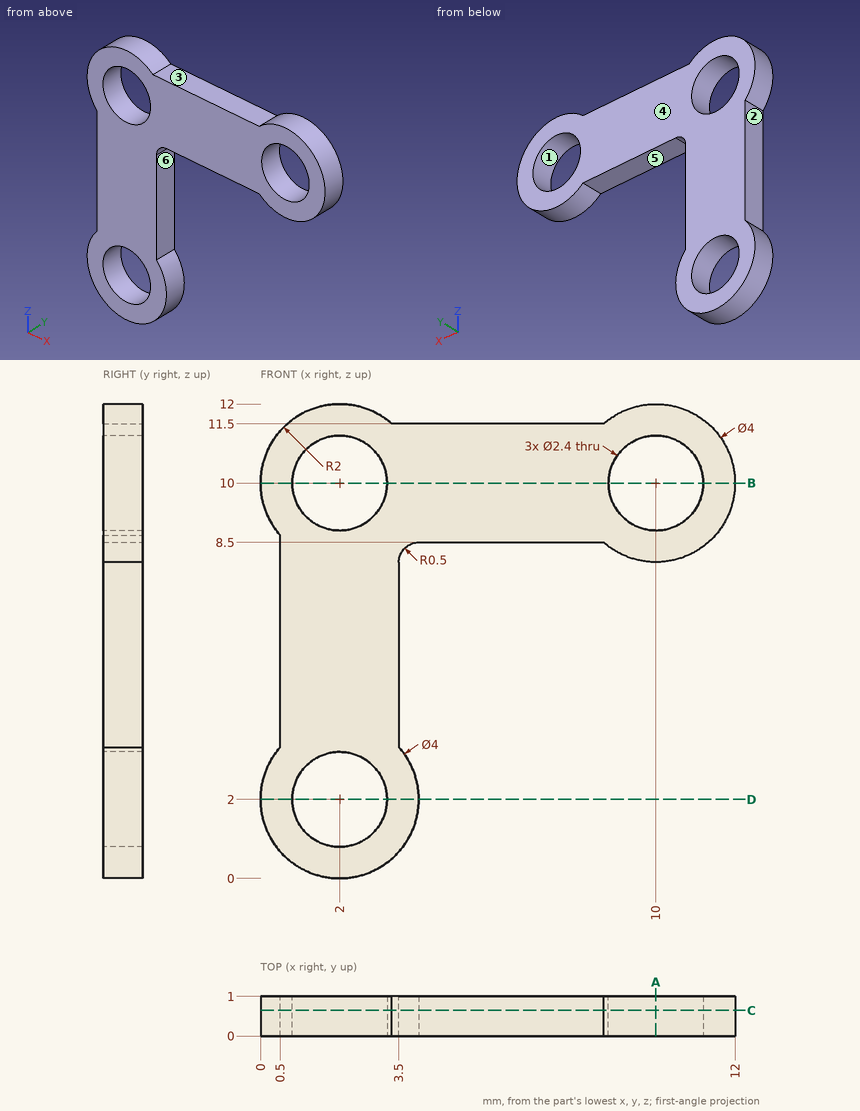
Geometry check sheet. Reference: drawing and pictorial views, mm from the part's lowest x, y, z. A direction names the side the tool comes from. Round coordinates to 2 decimals unless told otherwise and drop trailing zeros. Order: outer loops, then holes, each group sorted by start corner. A loop starts at its lowest first (then second) coordinate and runs counter-clockwise, first axis right, second up. Notation, with made-up numbers: M -21,-13 L -3,-13 A14 ccw -3,-8 Z; hole C 19.5,-1 d3. An arc over 180 degrees is marked long. Answer as CSV lines item,"result".
1) Gauge pin test, flat ends, axial feed: pin 1 Ø3 at (x, z) = (2, 2) entering from -Y; pin 2 Ø2 at (x, z) = (10, 10) entering from +Y. Record the tip position at first contact, or that the pin passes through.
Entries:
pin 1,"y = 0"
pin 2,"through"
2) Tool access check on the marked faces 1, 2 and 3. Record the directions out of +Z, -Z, +X, -X, +Y, -Y that give a thin tool (end or side, any length) a straight path to the whole face; none if there is none.
Entries:
face 1,"+Y, -Y"
face 2,"-X, +Y, -Y"
face 3,"+Z, +Y, -Y"
3) Sectioned sample at C-C on y = 0.65. Record the cut outline in (x, z).
Entries:
outline,"M 0.5,3.32 A2 ccw long 3.5,3.32 L 3.5,8 A0.5 cw 4,8.5 L 8.68,8.5 A2 ccw long 8.68,11.5 L 3.32,11.5 A2 ccw 0.5,8.68 Z; hole C 2,2 d2.4; hole C 2,10 d2.4; hole C 10,10 d2.4"
4) Thickness scan on probe 1 along Z at (x, y) = (2, 0.65); probe 2 along Z at (x, y) = (10, 0.4). Record the ranges inside material, lowest first. Write a range as [from, to].
Entries:
probe 1,"[0, 0.8], [3.2, 8.8], [11.2, 12]"
probe 2,"[8, 8.8], [11.2, 12]"
5) Sectioned sample at B-B on z = 10. Record the cut outline in (x, y), and give its area (3 significant figures).
Entries:
outline,"M 0,0 L 0.8,0 L 0.8,1 L 0,1 Z; M 3.2,0 L 8.8,0 L 8.8,1 L 3.2,1 Z; M 11.2,0 L 12,0 L 12,1 L 11.2,1 Z"
area,"7.20 mm2"
6) Sectioned sample at A-A on x = 10. Record the cut outline in (y, z).
Entries:
outline,"M 0,8 L 1,8 L 1,8.8 L 0,8.8 Z; M 0,11.2 L 1,11.2 L 1,12 L 0,12 Z"
7) Sectioned sample at D-D on z = 2. Record the cut outline in (x, y).
Entries:
outline,"M 0,0 L 0.8,0 L 0.8,1 L 0,1 Z; M 3.2,0 L 4,0 L 4,1 L 3.2,1 Z"
8) Mould release check, pull along X, two halves, no side actions. Record for the marked faces 4, 5 and 6: +X half, -X half, draft (parallel to the pull), parting line (faces both ways), or undercut.
Entries:
face 4,"draft"
face 5,"undercut"
face 6,"+X half"
